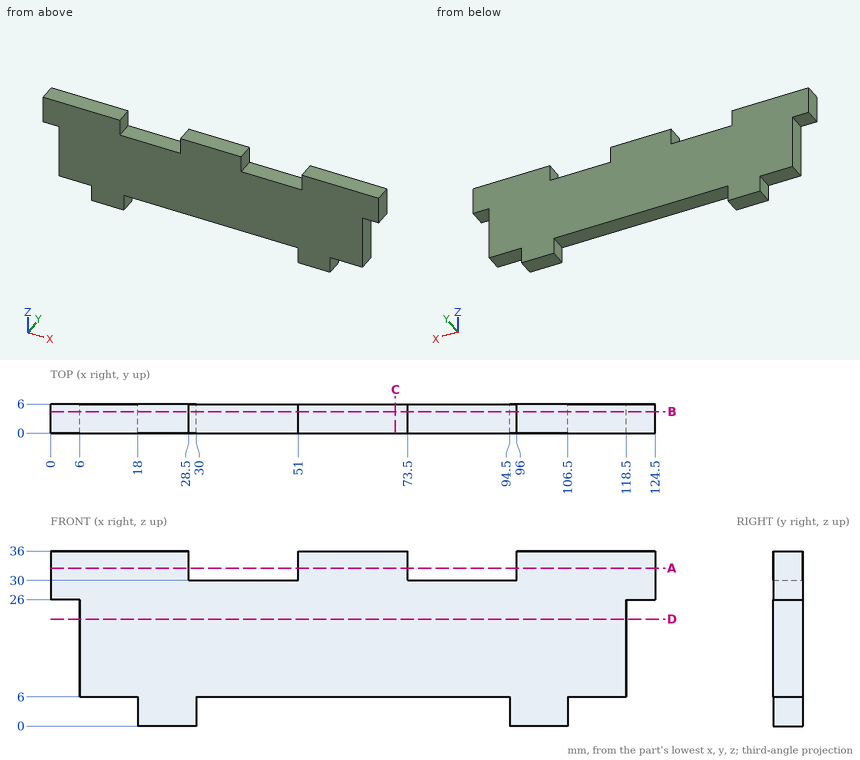
Source: three-view drawing plus pictorial views. Frame: mm from the lowest corner of the part. Give positions to 0.01 mm unless a question says otherwise; leave off trailing zeros. Loops run counter-clockwise (first coordinate to the right, second up) from the corner with the lowest first, then second, coordinate; pieces in that order, holes last. Notation, with made-up numbers: M -8,78 L 12,78 A23 cw 12,93 Z; hole C -24,-34.75 d5. An arc over 180 degrees is marked long. Put each result on its own line as item: value.
Q1. Section A-A (z = 32.5). Return the cut outline in (x, y).
Response values:
outline: M 0,0 L 28.5,0 L 28.5,6 L 0,6 Z; M 51,0 L 73.5,0 L 73.5,6 L 51,6 Z; M 96,0 L 124.5,0 L 124.5,6 L 96,6 Z
Q2. Pin query (flat end, axial travel): P1, Ø3, axis at x = 110.5, y = 2, coming from the -Z side; P2, Ø3, axis at x = 67.5, z = 5, coming from the +Y side; P3, Ø2, axis at y = 3.5, z = 20, coming from the -X side; P4, Ø1.8, axis at x = 4, y = 1.5, coming from the -Z side. Return the tip coordinate at first contact, or that it passes through.
Response values:
P1: stops at z = 6
P2: stops at y = 6
P3: stops at x = 6
P4: stops at z = 26
Q3. Line query: probe 1 along X at (y, z) = (4.1, 4.5); probe 2 along X at (y, z) = (1.65, 33.5); probe 3 along X at (y, z) = (5.05, 13). Output: solid intervals per line, ascending. Write a range as [from, to].
Response values:
probe 1: x = [18, 30], [94.5, 106.5]
probe 2: x = [0, 28.5], [51, 73.5], [96, 124.5]
probe 3: x = [6, 118.5]
Q4. Section C-C (x = 71). Return the cut outline in (y, z), and give its area (3 significant figures).
Response values:
outline: M 0,6 L 6,6 L 6,36 L 0,36 Z
area: 180 mm²
Q5. Section D-D (z = 22). Return the cut outline in (x, y), and give its area (3 significant figures).
Response values:
outline: M 6,0 L 118.5,0 L 118.5,6 L 6,6 Z
area: 675 mm²
Q6. Section B-B (y = 4.45). Return the cut outline in (x, z), and give its area (3 significant figures).
Response values:
outline: M 0,26 L 6,26 L 6,6 L 18,6 L 18,0 L 30,0 L 30,6 L 94.5,6 L 94.5,0 L 106.5,0 L 106.5,6 L 118.5,6 L 118.5,26 L 124.5,26 L 124.5,36 L 96,36 L 96,30 L 73.5,30 L 73.5,36 L 51,36 L 51,30 L 28.5,30 L 28.5,36 L 0,36 Z
area: 3,370 mm²
